Part model, mm, in its own coordinate system. A direction names the side the tool comes from. Round coordinates to 2 decimals unless told otherwise and drop trailing zeros. Write each loop counter-clockwise with the first axis right and the second up, starting at its lowest first coordinate (ties: lowest second). Pieces come first, ordered by that corner, then holes. Notation, with made-up numbers: (87.5, 86.5) -> (96.5, 86.5) arc R33 cw to (96.5, 116.5) -> close; hole circle Ø6 at (55.25, 53.5). An arc over 180 degrees is marked (long way). Return JSON: item names as keys, results as strings. Group by question number.
```python
from build123d import *

# Parameters (mm, degrees)
F1_DEPTH = 127
F2_W     = 42.6925110772
F2_H     = 83.2166295946
F3_DEPTH = 25.4
F4_W     = 42.6925110772
F4_H     = 41.6083147973
F5_DEPTH = 12.7


with BuildPart() as f1:
    # F0 (on Top) → F1 (new body)
    with BuildSketch(Plane.XY):
        Polygon((15.3271912833, 67.492875863), (-10.8187645674, 72.8341937065), (31.1941243708, -20.2240943909), (50.9100646707, -11.32296772), align=None)
    extrude(amount=F1_DEPTH)

    # F2 (on face) → F3 (join)
    with BuildSketch(Plane(origin=(18.3279159537, 8.2744773537, 0), x_dir=(0.4114774291, -0.9114199501, 0), z_dir=(-0.9114199501, -0.4114774291, 0))):
        with Locations((-11.9696195438, 63.5)):
            Rectangle(F2_W, F2_H)
    extrude(amount=F3_DEPTH)

    # F4 (on face) → F5 (join)
    with BuildSketch(Plane(origin=(-4.822150778, -2.1770493443, 0), x_dir=(0.4114774291, -0.9114199501, 0), z_dir=(-0.9114199501, -0.4114774291, 0))):
        with Locations((-11.9696195438, 42.6958426014)):
            Rectangle(F4_W, F4_H)
    extrude(amount=F5_DEPTH)


solid = f1.part
```
Item 1: Wall check: L1, parallel to Z at x = -5, y = 18.5; L2, parallel to X at y = 22, z = 28.5; L3, parallel to X at y = 20, z = 45. Give the ranges that are in metal, low to high.
Item 2: Flat gauge pins, fed straight in: P1, Ø3, axis at x = -10, y = 0.5, coming from the +Z side; P2, Ø20.5, axis at x = -6, y = 2.5, coming from the +Z side; P3, Ø1.5, axis at y = 62.5, z = 24, coming from the +X side. Where does each tip first touch, or does it go through?
Item 3: Cut at C-C (x = 20). Write the cut outline in (y, z).
Item 4: Cut at B-B (z = 101.5). Write the cut outline in (x, y), then the cut area to 3 significant figures.
Item 5: Cut at D-D (y = 4.5). Write the cut outline in (x, z), then the cut area to 3 significant figures.
Item 6: Which spindle directions (+Z, -Z, +X, -X, +Y, -Y) get a long thin tool onto all of the face, cutting with end or side? Do faces 1 (the face through (-4, 12, 21.892)), 2 (the face through (-9.87, 9, 84.6)), 3 (the face through (20, 27, 127)). Say none if no direction does.
Item 7: Two-plate mould, pull along X, no slides. Class faces 4 (the face through (-16, 6, 63.5)), 5 (the face through (8.925, -6.259, 62.917)), 6 (the face through (-8.642, 32.652, 62.917)): released by +X, released by -X, zero draft, split by the parting line, or undercut.
Item 8: Cut at A-A (x = -6.5). Write the cut outline in (y, z), then the cut area to 3 significant figures.
Checks:
{
 "1": {"L1": "z = 21.89 to 105.11", "L2": "x = -29.67 to 35.87", "L3": "x = -28.77 to 36.77"},
 "2": {"P1": "stops at z = 63.5", "P2": "stops at z = 105.11", "P3": "stops at x = 17.92"},
 "3": {"outline": "(-1.26, 21.89) -> (4.57, 21.89) -> (4.57, 0) -> (57.14, 0) -> (57.14, 127) -> (4.57, 127) -> (4.57, 105.11) -> (-1.26, 105.11) -> close"},
 "4": {"outline": "(-18.53, 28.19) -> (-0.96, -10.72) -> (22.19, -0.27) -> (31.19, -20.22) -> (50.91, -11.32) -> (15.33, 67.49) -> (-10.82, 72.83) -> (4.62, 38.64) -> close", "area": "3,120 mm2"},
 "5": {"outline": "(-21.77, 21.89) -> (20.03, 21.89) -> (20.03, 0) -> (43.77, 0) -> (43.77, 127) -> (20.03, 127) -> (20.03, 105.11) -> (-7.84, 105.11) -> (-7.84, 63.5) -> (-21.77, 63.5) -> close", "area": "5,910 mm2"},
 "6": {"face 1": "-Z, -X, -Y", "face 2": "+Z, -X, -Y", "face 3": "+Z, +X, -X, +Y, -Y"},
 "7": {"face 4": "zero draft", "face 5": "undercut", "face 6": "released by -X"},
 "8": {"outline": "(-13.22, 21.89) -> (33.62, 21.89) -> (33.62, 105.11) -> (1.54, 105.11) -> (1.54, 63.5) -> (-13.22, 63.5) -> close; (63.27, 0) -> (71.95, 0) -> (71.95, 127) -> (63.27, 127) -> close", "area": "4,390 mm2"}
}
